```python
from build123d import *

# Parameters (mm, degrees)
SKETCH1_R           = 18
BOSS_EXTRUDE1_DEPTH = 4
CUT_EXTRUDE1_REACH  = 178.366
SKETCH2_R           = 1.5
BOSS_EXTRUDE2_START = 27
BOSS_EXTRUDE2_DEPTH = 27
SKETCH4_W           = 86
SKETCH4_H           = 60
BOSS_EXTRUDE5_DEPTH = 5
BOSS_EXTRUDE6_START = -31
BOSS_EXTRUDE6_DEPTH = 31
BOSS_EXTRUDE7_DEPTH = 27
SKETCH9_R           = 1.5
BOSS_EXTRUDE8_DEPTH = 3
FILLET2_R           = 5
FILLET3_R           = 1
CUT_EXTRUDE2_REACH  = 157.453
SKETCH10_R          = 2.5


with BuildPart() as part:
    # Sketch1 → Boss-Extrude1 (new body)
    with BuildSketch(Plane(origin=(0, 24.62645802, -24.62645802), x_dir=(1, 0, 0), z_dir=(2.4702462297909737e-15, -0.70710678118655, 0.707106781186545))):
        with Locations(Location((73.844609768, 130.551114539, 0), (0, 0, 90))):
            Circle(SKETCH1_R)
        with BuildLine():
            Line((83.2907778, 127.269360509), (77.126363797, 121.104946506))
            ThreePointArc((77.126363797, 121.104946506), (66.773541956, 123.480046727), (64.398441736, 133.832868568))
            Line((64.398441736, 133.832868568), (70.562855738, 139.997282571))
            ThreePointArc((70.562855738, 139.997282571), (80.91567758, 137.62218235), (83.2907778, 127.269360509))
        make_face(mode=Mode.SUBTRACT)
    extrude(amount=BOSS_EXTRUDE1_DEPTH)

    # Sketch2 → Cut-Extrude1 (cut, up to next)
    with BuildSketch(Plane(origin=(0, 24.62645802, -24.62645802), x_dir=(1, 0, 0), z_dir=(-2.4702462297909737e-15, 0.70710678118655, -0.707106781186545)), mode=Mode.PRIVATE) as cut_extrude1_sk1:
        with Locations(Location((86.844609768, -130.551114539, 0), (0, 0, 270))):
            Circle(SKETCH2_R)
    cut_extrude1_tool1 = extrude(cut_extrude1_sk1.sketch, amount=-CUT_EXTRUDE1_REACH, mode=Mode.PRIVATE) & part.part
    # Sketch2 → Cut-Extrude1 (cut, up to next)
    with BuildSketch(Plane(origin=(0, 24.62645802, -24.62645802), x_dir=(1, 0, 0), z_dir=(-2.4702462297909737e-15, 0.70710678118655, -0.707106781186545)), mode=Mode.PRIVATE) as cut_extrude1_sk2:
        with Locations(Location((73.844609768, -143.551114539, 0), (0, 0, 270))):
            Circle(SKETCH2_R)
    cut_extrude1_tool2 = extrude(cut_extrude1_sk2.sketch, amount=-CUT_EXTRUDE1_REACH, mode=Mode.PRIVATE) & part.part
    # Sketch2 → Cut-Extrude1 (cut, up to next)
    with BuildSketch(Plane(origin=(0, 24.62645802, -24.62645802), x_dir=(1, 0, 0), z_dir=(-2.4702462297909737e-15, 0.70710678118655, -0.707106781186545)), mode=Mode.PRIVATE) as cut_extrude1_sk3:
        with Locations(Location((60.844609768, -130.551114539, 0), (0, 0, 270))):
            Circle(SKETCH2_R)
    cut_extrude1_tool3 = extrude(cut_extrude1_sk3.sketch, amount=-CUT_EXTRUDE1_REACH, mode=Mode.PRIVATE) & part.part
    # Sketch2 → Cut-Extrude1 (cut, up to next)
    with BuildSketch(Plane(origin=(0, 24.62645802, -24.62645802), x_dir=(1, 0, 0), z_dir=(-2.4702462297909737e-15, 0.70710678118655, -0.707106781186545)), mode=Mode.PRIVATE) as cut_extrude1_sk4:
        with Locations(Location((73.844609768, -117.551114539, 0), (0, 0, 270))):
            Circle(SKETCH2_R)
    cut_extrude1_tool4 = extrude(cut_extrude1_sk4.sketch, amount=-CUT_EXTRUDE1_REACH, mode=Mode.PRIVATE) & part.part
    add(cut_extrude1_tool1.solids().sort_by_distance((86.84461, 116.940036, 67.68712))[0], mode=Mode.SUBTRACT)
    add(cut_extrude1_tool2.solids().sort_by_distance((73.84461, 126.132425, 76.879509))[0], mode=Mode.SUBTRACT)
    add(cut_extrude1_tool3.solids().sort_by_distance((60.84461, 116.940036, 67.68712))[0], mode=Mode.SUBTRACT)
    add(cut_extrude1_tool4.solids().sort_by_distance((73.84461, 107.747648, 58.494732))[0], mode=Mode.SUBTRACT)

    # Sketch3 → Boss-Extrude2 (add)
    with BuildSketch(Plane(origin=(0, 24.62645802, -24.62645802), x_dir=(1, 0, 0), z_dir=(-2.4702462297909737e-15, 0.70710678118655, -0.707106781186545)).offset(BOSS_EXTRUDE2_START)):
        with BuildLine():
            Line((91.844609768, -130.551114539), (89.844609768, -130.551114539))
            ThreePointArc((89.844609768, -130.551114539), (73.844609768, -114.551114539), (57.844609768, -130.551114539))
            Line((57.844609768, -130.551114539), (55.844609768, -130.551114539))
            ThreePointArc((55.844609768, -130.551114539), (73.844609768, -112.551114539), (91.844609768, -130.551114539))
        make_face()
    extrude(amount=-BOSS_EXTRUDE2_DEPTH)



with BuildPart() as body_2:
    # Sketch4 → Boss-Extrude5 (new body)
    with BuildSketch(Plane(origin=(0, 79.58565632, 79.58565632), x_dir=(-1, 0, 0), z_dir=(0, -0.7071067811865451, -0.70710678118655))):
        with Locations((-73.844609768, 60.827070924)):
            Rectangle(SKETCH4_W, SKETCH4_H)
    extrude(amount=BOSS_EXTRUDE5_DEPTH)


with BuildPart() as part_1:
    add(part.part)

    add(body_2.part)  # Boss-Extrude6 merges body 2
    # Sketch6 → Boss-Extrude6 (add)
    with BuildSketch(Plane(origin=(0, 21.798030895, -21.798030895), x_dir=(1, 0, 0), z_dir=(2.4702462297909737e-15, -0.70710678118655, 0.707106781186545)).offset(BOSS_EXTRUDE6_START)):
        with BuildLine():
            ThreePointArc((73.844609768, 112.551114539), (61.116687706, 117.823192477), (55.844609768, 130.551114539))
            Line((55.844609768, 130.551114539), (48.844609768, 112.551114539))
            Line((48.844609768, 112.551114539), (73.844609768, 112.551114539))
        make_face()
        with BuildLine():
            Line((57.844609768, 130.551114539), (55.844609768, 130.551114539))
            ThreePointArc((55.844609768, 130.551114539), (61.116687706, 117.823192477), (73.844609768, 112.551114539))
            ThreePointArc((73.844609768, 112.551114539), (86.572531829, 117.823192477), (91.844609768, 130.551114539))
            Line((91.844609768, 130.551114539), (89.844609768, 130.551114539))
            ThreePointArc((89.844609768, 130.551114539), (73.844609768, 114.551114539), (57.844609768, 130.551114539))
        make_face()
        with BuildLine():
            ThreePointArc((91.844609768, 130.551114539), (86.572531829, 117.823192477), (73.844609768, 112.551114539))
            Line((73.844609768, 112.551114539), (98.844609768, 112.551114539))
            Line((98.844609768, 112.551114539), (91.844609768, 130.551114539))
        make_face()
    extrude(amount=BOSS_EXTRUDE6_DEPTH)

    # Sketch8 → Boss-Extrude7 (add)
    with BuildSketch(Plane(origin=(0, 64.224437766, -64.224437766), x_dir=(1, 0, 0), z_dir=(0, 0.7071067811865498, -0.7071067811865452))):
        with BuildLine():
            Line((91.844609768, -130.551114539), (88.844609768, -130.551114539))
            ThreePointArc((88.844609768, -130.551114539), (73.844609768, -115.551114539), (58.844609768, -130.551114539))
            Line((58.844609768, -130.551114539), (55.844609768, -130.551114539))
            Line((55.844609768, -130.551114539), (55.844609768, -112.551114539))
            Line((55.844609768, -112.551114539), (91.844609768, -112.551114539))
            Line((91.844609768, -112.551114539), (91.844609768, -130.551114539))
        make_face()
    extrude(amount=-BOSS_EXTRUDE7_DEPTH)

    # Sketch9 → Boss-Extrude8 (add)
    # profile 1 of 2: a face of its own
    with BuildSketch(Plane(origin=(0, 92.313578382, 92.313578382), x_dir=(1, 0, 0), z_dir=(-6.542051911181989e-15, 0.7071067811865454, 0.7071067811865497))):
        with BuildLine():
            Line((55.844609768, 72.327070924), (49.919173765, 73.951634922))
            ThreePointArc((49.919173765, 73.951634922), (47.344609768, 77.327070924), (49.919173765, 80.702506927))
            Line((49.919173765, 80.702506927), (55.844609768, 82.327070924))
            Line((55.844609768, 82.327070924), (55.844609768, 72.327070924))
        make_face()
        with Locations(Location((50.844609768, 77.327070924, 0), (0, 0, 270))):
            Circle(SKETCH9_R, mode=Mode.SUBTRACT)
    # profile 2 of 2: a face of its own
    with BuildSketch(Plane(origin=(0, 92.313578382, 92.313578382), x_dir=(1, 0, 0), z_dir=(-6.542051911181989e-15, 0.7071067811865454, 0.7071067811865497))):
        with BuildLine():
            Line((97.77004577, 80.702506927), (91.844609768, 82.327070924))
            Line((91.844609768, 82.327070924), (91.844609768, 72.327070924))
            Line((91.844609768, 72.327070924), (97.77004577, 73.951634922))
            ThreePointArc((97.77004577, 73.951634922), (100.344609768, 77.327070924), (97.77004577, 80.702506927))
        make_face()
        with Locations(Location((96.844609768, 77.327070924, 0), (0, 0, 270))):
            Circle(SKETCH9_R, mode=Mode.SUBTRACT)
    extrude(amount=-BOSS_EXTRUDE8_DEPTH)

    # Fillet2
    fillet2_edges = [part_1.edges().sort_by_distance(p)[0] for p in [
        (98.844609768, 112.343842324, 46.827470317),
        (48.844609768, 112.343842324, 46.827470317),
        (30.844609768, 99.615920262, 56.019858473),
        (30.844609768, 142.042327133, 13.593451601),
        (116.844609768, 142.042327133, 13.593451601),
        (116.844609768, 99.615920262, 56.019858473),
        (91.844609768, 134.26415254, 24.9071601),
        (55.844609768, 134.26415254, 24.9071601),
    ]]
    fillet(fillet2_edges, radius=FILLET2_R)

    # Fillet3
    fillet3_edges = [part_1.edges().sort_by_distance(p)[0] for p in [
        (55.844609768, 144.870754258, 35.513761818),
        (91.844609768, 144.870754258, 35.513761818),
    ]]
    fillet(fillet3_edges, radius=FILLET3_R)

    # Sketch10 → Cut-Extrude2 (cut, up to next)
    with BuildSketch(Plane(origin=(0, 79.58565632, 79.58565632), x_dir=(1, 0, 0), z_dir=(0, 0.7071067811865451, 0.70710678118655)), mode=Mode.PRIVATE) as cut_extrude2_sk1:
        with Locations(Location((108.844609768, 40.827070924, 0), (0, 0, 270))):
            Circle(SKETCH10_R)
    cut_extrude2_tool1 = extrude(cut_extrude2_sk1.sketch, amount=-CUT_EXTRUDE2_REACH, mode=Mode.PRIVATE) & part_1.part
    # Sketch10 → Cut-Extrude2 (cut, up to next)
    with BuildSketch(Plane(origin=(0, 79.58565632, 79.58565632), x_dir=(1, 0, 0), z_dir=(0, 0.7071067811865451, 0.70710678118655)), mode=Mode.PRIVATE) as cut_extrude2_sk2:
        with Locations(Location((38.844609768, 40.827070924, 0), (0, 0, 270))):
            Circle(SKETCH10_R)
    cut_extrude2_tool2 = extrude(cut_extrude2_sk2.sketch, amount=-CUT_EXTRUDE2_REACH, mode=Mode.PRIVATE) & part_1.part
    # Sketch10 → Cut-Extrude2 (cut, up to next)
    with BuildSketch(Plane(origin=(0, 79.58565632, 79.58565632), x_dir=(1, 0, 0), z_dir=(0, 0.7071067811865451, 0.70710678118655)), mode=Mode.PRIVATE) as cut_extrude2_sk3:
        with Locations(Location((108.844609768, 60.827070924, 0), (0, 0, 270))):
            Circle(SKETCH10_R)
    cut_extrude2_tool3 = extrude(cut_extrude2_sk3.sketch, amount=-CUT_EXTRUDE2_REACH, mode=Mode.PRIVATE) & part_1.part
    # Sketch10 → Cut-Extrude2 (cut, up to next)
    with BuildSketch(Plane(origin=(0, 79.58565632, 79.58565632), x_dir=(1, 0, 0), z_dir=(0, 0.7071067811865451, 0.70710678118655)), mode=Mode.PRIVATE) as cut_extrude2_sk4:
        with Locations(Location((38.844609768, 60.827070924, 0), (0, 0, 270))):
            Circle(SKETCH10_R)
    cut_extrude2_tool4 = extrude(cut_extrude2_sk4.sketch, amount=-CUT_EXTRUDE2_REACH, mode=Mode.PRIVATE) & part_1.part
    add(cut_extrude2_tool1.solids().sort_by_distance((108.84461, 108.454755, 50.716558))[0], mode=Mode.SUBTRACT)
    add(cut_extrude2_tool2.solids().sort_by_distance((38.84461, 108.454755, 50.716558))[0], mode=Mode.SUBTRACT)
    add(cut_extrude2_tool3.solids().sort_by_distance((108.84461, 122.596891, 36.574422))[0], mode=Mode.SUBTRACT)
    add(cut_extrude2_tool4.solids().sort_by_distance((38.84461, 122.596891, 36.574422))[0], mode=Mode.SUBTRACT)


solid = part_1.part
```
Source: CAD feature listing. Evaluate the final solid. Frame: model axes, mm. A direction names the side the tool comes from. Give positions to 0.01 mm unless a question says otherwise; leave off trailing zeros. Put each result on its own line as item: value. Start each with the question number.
1) Draft query along Y for faces 1 (the face through (116.845, 121, 35)), 2 (the face through (40.95, 119.9, 35.78)), 3 (the face through (52.814, 144.918, 35.467)), 4 (the face through (115.34, 100.6, 54.99)). Return one class per face: released by +Y, released by -Y, zero draft, split by the parting line, or undercut.
2) Contact query for flat-ended pins moving along their axis: P1, Ø8, axis at x = 74, z = 52, coming from the +Y side; P2, Ø1.5, axis at x = 83, y = 137, coming from the -Z side; P3, Ø4, axis at x = 98, y = 110, coming from the -Z side. Output: stop coordinate, or through.
3) Material intervals for probe 1 along Y at (x, z) = (74, 35); probe 2 along Y at (x, z) = (35, 38.5); probe 3 along Z at (x, y) = (43, 104), sorted ascending.
4) Reachability of faces 5 (the face through (80.252, 111.076, 64.612)), 6 (the face through (93.348, 135.139, 26.049)), 7 (the face through (74.167, 125.336, 35.071)) from +Z, -Z, +X, -X, +Y, -Y: full face, straight path, thin tool, end or side. Return the list, or none.
5) Cut plane A-A (z = 44). State how many separate pieces and enclosed holes the cut face has, then the cut area to 3 significant figures.
Results are:
1. face 1: zero draft
1. face 2: undercut
1. face 3: undercut
1. face 4: released by -Y
2. P1: stops at y = 114
2. P2: stops at z = 14.35
2. P3: stops at z = 40.1
3. probe 1: y = 117.1 to 124.17, 125.27 to 128.42
3. probe 2: y = 113.6 to 120.67
3. probe 3: z = 48.1 to 55.17
4. face 5: +Z, +Y
4. face 6: +X
4. face 7: +X, -X
5. separate pieces: 3
5. enclosed holes: 0
5. area: 1,110 mm2
